Part model, mm, in its own coordinate system. Round coordinates to 2 decimals unless told otherwise and drop trailing zeros. Write each loop counter-clockwise with the first axis right and the second up, starting at its lowest first coordinate (ties: lowest second). Pieces come first, ordered by that corner, then holes. Notation, with made-up numbers: (-27, -37) -> (14, -37) arc R28 ccw to (14, -13) -> close; hole circle Ø1 at (48.25, 75). An arc over 180 degrees is marked (long way). Return JSON: item names as keys, results as strings. Group by question number.
(1) Saw through at C-C (z = 1.8). State how many separate pieces and enclosed holes the cut face has, plus the area to 3 significant figures.
(2) Drill centre lines: L1, parallel to X at y = -8.25, z = 2.7; L2, parallel to Y at x = 39, z = 4. Where is each one in solid material? Low to high. Write a range as from..to.
(3) Drop flat-ended pins along their axis: pin 1 Ø3 at (y, z) = (-6, 4) entering from -X; pin 2 Ø3 at (x, z) = (26.5, 4) entering from -Y; pin 3 Ø0.7 at (y, z) = (-5, 3) entering from -X. Give the stop position or say it passes through.
(4) Saw through at A-A (y = 0). List the corners of the cut face in (x, z), plus the area to 4 significant figures.
(5) Saw through at B-B (x = 26). List the corners of the cut face in (y, z).
from build123d import *

# Parameters (mm, degrees)
F0_W     = 3.175
F0_H     = 3.175
F1_DEPTH = 6


with BuildPart() as f1:
    # F0 (on Top) → F1 (new body)
    with BuildSketch(Plane.XY):
        with BuildLine():
            ThreePointArc((269.931261, -7.9375), (277.868761, 0), (269.931261, 7.9375))
            Line((269.931261, 7.9375), (0, 7.9375))
            ThreePointArc((0, 7.9375), (-7.9375, 0), (0, -7.9375))
            Line((0, -7.9375), (93.662513, -7.9375))
            Line((93.662513, -7.9375), (93.662513, -10.31875))
            Line((93.662513, -10.31875), (100.012513, -10.31875))
            Line((100.012513, -10.31875), (100.012513, -3.96875))
            Line((100.012513, -3.96875), (93.662513, -3.96875))
            Line((93.662513, -3.96875), (93.662513, -6.35))
            Line((93.662513, -6.35), (0, -6.35))
            ThreePointArc((0, -6.35), (-6.35, 0), (0, 6.35))
            Line((0, 6.35), (269.931261, 6.35))
            ThreePointArc((269.931261, 6.35), (276.281261, 0), (269.931261, -6.35))
            Line((269.931261, -6.35), (176.268748, -6.35))
            Line((176.268748, -6.35), (176.268748, -3.96875))
            Line((176.268748, -3.96875), (173.093748, -3.96875))
            Line((173.093748, -3.96875), (169.918748, -3.96875))
            Line((169.918748, -3.96875), (169.918748, -10.31875))
            Line((169.918748, -10.31875), (176.268748, -10.31875))
            Line((176.268748, -10.31875), (176.268748, -7.9375))
            Line((176.268748, -7.9375), (269.931261, -7.9375))
        make_face()
        with Locations((96.837513, -7.14375)):
            Rectangle(F0_W, F0_H, mode=Mode.SUBTRACT)
        Polygon((171.506248, -5.55625), (173.093748, -5.55625), (174.681248, -5.55625), (174.681248, -8.73125), (171.506248, -8.73125), align=None, mode=Mode.SUBTRACT)
    extrude(amount=F1_DEPTH)


solid = f1.part
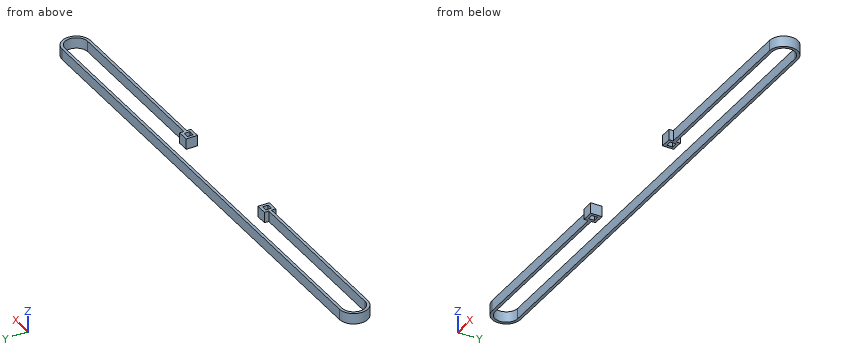
Computed values:
{
 "1": {"separate pieces": "1", "enclosed holes": "2", "area": "858 mm2"},
 "2": {"L1": "93.66..95.25, 98.43..100.01, 169.92..171.51, 174.68..176.27", "L2": "-7.94..-6.35, 6.35..7.94"},
 "3": {"pin 1": "x = -6.54", "pin 2": "y = -7.94", "pin 3": "x = -6.43"},
 "4": {"outline": "(-7.94, 0) -> (-6.35, 0) -> (-6.35, 6) -> (-7.94, 6) -> close; (276.28, 0) -> (277.87, 0) -> (277.87, 6) -> (276.28, 6) -> close", "area": "19.05 mm2"},
 "5": {"outline": "(-7.94, 0) -> (-6.35, 0) -> (-6.35, 6) -> (-7.94, 6) -> close; (6.35, 0) -> (7.94, 0) -> (7.94, 6) -> (6.35, 6) -> close"}
}
